Input: part model. Units: mm. Frame: model coordinates. A direction names the side the tool comes from. Round coordinates to 2 decimals unless told otherwise and drop trailing zeros. Loops run counter-clockwise (first coordinate to the right, second up) from the corner with the lowest first, then second, coordinate; pieces in that order, holes last. Notation, with made-up numbers: M -2,17.5 L 21,17.5 A5 ccw 21,24.5 Z; hole C 37,-39.5 d6. An arc over 180 degrees is marked long. Use one line per item in the form item = value. Start each with the question number.
Q1. First-contact query: P1, Ø4.5, axis at y = -106, z = 6, coming from the +X side; P2, Ø6.5, axis at x = 27, z = 9, coming from the -Y side; P3, Ø5.5, axis at x = -22.86, z = 5.08, coming from the -Y side; P4, Ø1.8, axis at y = -15.88, z = 6.35, coming from the +X side. Flat tips, straight axial feed; report the tip coordinate or a pass-through.
Q2. Ray query, line 1 along Y through (x, z) = (0, 9.75) (1 decimal); line 2 along X through (y, z) = (-15.5, 2.5); line 3 along Y through (x, z) = (-33, 10) (3 decimals). Return the intervals inside material, ascending.
Q3. Section query A-A, the plane x = 0. Output: boundary loops of the cut face in (y, z) (1 decimal), and give its area (3 significant figures).
Q4. Section query D-D, the plane x = 43. Output: boundary loops of the cut face in (y, z) (3 decimals), and give its area (3 significant figures).
Q5. Access query for faces 1 (the flat face through (10.16, -106, 6)), 2 (the flat face through (15, -3.175, 7)), 3 (the flat face through (32.166, -73.576, 6.261)). Directions: +Z, -Z, +X, -X, +Y, -Y. A direction counts if a zero-diameter tool reaches every point of the face in a straight line with its end or side. Return the directions, or none.
Q6. Section query C-C, the plane y = -106.5. Output: boundary loops of the cut face in (x, z), and give its area (3 significant figures).
Q7. Mould query, pull axis Y, two halves, no side actions, for faces 4 (the flat face through (-22.526, -64.63, 6.261)), 5 (the flat face through (-15, -3.175, 6)), 6 (the cylindrical face through (-19.32, 0.04, 7.44)), 7 (the flat face through (-31.64, -72.42, 6.26)). Classes: pulls with the +Y half, pulls with the -Y half, needs draft (parallel to the pull), parting line crosses it, or undercut.
Q8. Section query B-B, the plane x = 22. State how many separate pieces and enclosed holes the cut face has, and give its area (3 significant figures).
```python
from build123d import *

# Parameters (mm, degrees)
SKETCH3_R               = 9.5885
BOSS_EXTRUDE1_DEPTH     = 12.7
SKETCH4_R               = 3.614257139
CUT_EXTRUDE1_DEPTH      = 6.35
CUT_EXTRUDE2_START      = -12.7
CUT_EXTRUDE2_OUTLINE_R  = 1.5
CUT_EXTRUDE2_DEPTH      = 25.4
CUT_EXTRUDE3_DEPTH      = 126.664030474
CUT_EXTRUDE3_DEPTH_BACK = 126.664030474
SKETCH8_W               = 25.4
SKETCH8_H               = 5.08
SKETCH9_R               = 3
CUT_EXTRUDE4_DEPTH      = 123.783240632


# Read off the part's stored shape, not the designer's step: Cut-Extrude2
with BuildPart() as part:
    # Sketch3 → Boss-Extrude1 (new body)
    with BuildSketch(Plane.XY):
        with BuildLine():
            Line((50.652428891, 3.175), (-50.652428891, 3.175))
            Line((-50.652428891, 3.175), (-50.652428891, -3.175))
            Line((-50.652428891, -3.175), (-17.78, -3.175))
            ThreePointArc((-17.78, -3.175), (-14.187897552, -4.662897552), (-12.7, -8.255))
            Line((-12.7, -8.255), (-12.7, -29.595434395))
            ThreePointArc((-12.7, -29.595434395), (-12.814872576, -30.66963627), (-13.154295145, -31.69525691))
            Line((-13.154295145, -31.69525691), (-50.652428891, -114.3))
            Line((-50.652428891, -114.3), (-31.75, -114.3))
            Line((-31.75, -114.3), (-31.75, -109.5375))
            Line((-31.75, -109.5375), (31.75, -109.5375))
            Line((31.75, -109.5375), (31.75, -114.3))
            Line((31.75, -114.3), (50.652428891, -114.3))
            Line((50.652428891, -114.3), (13.154295145, -31.69525691))
            ThreePointArc((13.154295145, -31.69525691), (12.814872576, -30.66963627), (12.7, -29.595434395))
            Line((12.7, -29.595434395), (12.7, -8.255))
            ThreePointArc((12.7, -8.255), (14.187897552, -4.662897552), (17.78, -3.175))
            Line((17.78, -3.175), (50.652428891, -3.175))
            Line((50.652428891, -3.175), (50.652428891, 3.175))
        make_face()
        with Locations((0, -15.875)):
            Circle(SKETCH3_R, mode=Mode.SUBTRACT)
        with BuildLine():
            Line((-7.97501727, -32.575611881), (-37.490421301, -97.595177486))
            ThreePointArc((-37.490421301, -97.595177486), (-37.135167146, -102.446299841), (-32.864716446, -104.775))
            Line((-32.864716446, -104.775), (0, -104.775))
            Line((0, -104.775), (32.864716446, -104.775))
            ThreePointArc((32.864716446, -104.775), (37.135167146, -102.446299841), (37.490421301, -97.595177486))
            Line((37.490421301, -97.595177486), (7.97501727, -32.575611881))
            ThreePointArc((7.97501727, -32.575611881), (6.100612256, -30.404983695), (3.349312415, -29.595434395))
            Line((3.349312415, -29.595434395), (-3.349312415, -29.595434395))
            ThreePointArc((-3.349312415, -29.595434395), (-6.100612256, -30.404983695), (-7.97501727, -32.575611881))
        make_face(mode=Mode.SUBTRACT)
    extrude(amount=BOSS_EXTRUDE1_DEPTH)

    # Sketch4 → Cut-Extrude1 (cut)
    with BuildSketch(Plane(origin=(0, 3.175, 0), x_dir=(1, 0, 0), z_dir=(0, 1, 0))):
        with Locations(Location((-15.875, -6.35, 0), (0, 0, 180))):
            Circle(SKETCH4_R)
        with Locations(Location((15.875, -6.35, 0), (0, 0, 301.808324175))):
            Circle(SKETCH4_R)
    extrude(amount=-CUT_EXTRUDE1_DEPTH, mode=Mode.SUBTRACT)

    # Cut-Extrude2 outline → Cut-Extrude2 (cut)
    with BuildSketch(Plane.YZ.offset(CUT_EXTRUDE2_START)):
        with Locations((-15.883331584, 6.35)):
            Circle(CUT_EXTRUDE2_OUTLINE_R)
    extrude(amount=CUT_EXTRUDE2_DEPTH, mode=Mode.SUBTRACT)

    # Sketch8 → Cut-Extrude3 (cut, two sides: drawn at the far end of the back side and taken through both)
    with BuildSketch(Plane.XY.offset(12.7).offset(-CUT_EXTRUDE3_DEPTH_BACK)):
        with Locations((-22.86, -105.41)):
            Rectangle(SKETCH8_W, SKETCH8_H)
        with Locations((22.86, -105.41)):
            Rectangle(SKETCH8_W, SKETCH8_H)
    extrude(amount=CUT_EXTRUDE3_DEPTH + CUT_EXTRUDE3_DEPTH_BACK, mode=Mode.SUBTRACT)

    # Sketch9 → Cut-Extrude4 (cut, through all)
    with BuildSketch(Plane(origin=(0, -107.95, 0), x_dir=(1, 0, 0), z_dir=(0, 1, 0))):
        with Locations(Location((-22.86, -5.08, 0), (0, 0, 270))):
            Circle(SKETCH9_R)
        with Locations((22.86, -5.08)):
            Circle(SKETCH9_R)
    extrude(amount=-CUT_EXTRUDE4_DEPTH, mode=Mode.SUBTRACT)


solid = part.part
```
Results found:
q1.P1 = 47.91
q1.P2 = -109.54
q1.P3 = -71.42
q1.P4 = through
q2.line_1 = -109.5 to -104.8, -29.6 to -25.5, -6.3 to 3.2
q2.line_2 = -12.7 to -9.58, 9.58 to 12.7
q2.line_3 = -114.3 to -107.95, -87.703 to -75.413, -3.175 to 3.175
q3.outline = M -109.5,0 L -104.8,0 L -104.8,12.7 L -109.5,12.7 Z; M -29.6,0 L -25.5,0 L -25.5,12.7 L -29.6,12.7 Z; M -6.3,0 L 3.2,0 L 3.2,12.7 L -6.3,12.7 Z
q3.area = 233 mm²
q4.outline = M -114.3,0 L -97.442,0 L -97.442,12.7 L -114.3,12.7 Z; M -3.175,0 L 3.175,0 L 3.175,12.7 L -3.175,12.7 Z
q4.area = 295 mm²
q5.face_1 = +Z, -Z
q5.face_2 = +Y
q5.face_3 = +Z, -Z, +X
q6.outline = M -47.11,0 L -35.56,0 L -35.56,12.7 L -47.11,12.7 Z; M -10.16,0 L 10.16,0 L 10.16,12.7 L -10.16,12.7 Z; M 35.56,0 L 47.11,0 L 47.11,12.7 L 35.56,12.7 Z
q6.area = 551 mm²
q7.face_4 = undercut
q7.face_5 = pulls with the +Y half
q7.face_6 = needs draft
q7.face_7 = undercut
q8.separate_pieces = 4
q8.enclosed_holes = 0
q8.area = 248 mm²
